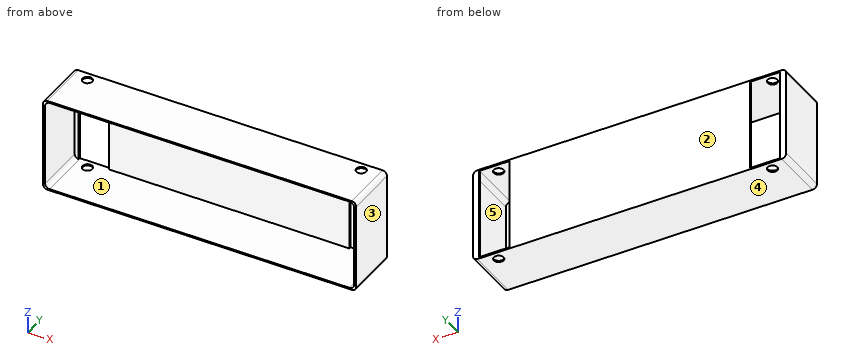
from build123d import *

# Parameters (mm, degrees)
SALIENTE_EXTRUIR1_DEPTH = 60
CROQUIS3_W              = 268.6
CROQUIS3_H              = 105
SALIENTE_EXTRUIR4_DEPTH = 2.4
CROQUIS4_R              = 5.5
CORTAR_EXTRUIR1_DEPTH   = 106


with BuildPart() as part:
    # Croquis2 → Saliente-Extruir1 (new body)
    with BuildSketch(Plane(origin=(0, 0, 0), x_dir=(1, 0, 0), z_dir=(0, 1, 0))):
        with BuildLine():
            Line((-170, 52.5), (170, 52.5))
            ThreePointArc((170, 52.5), (173.535533906, 51.035533906), (175, 47.5))
            Line((175, 47.5), (175, -47.5))
            ThreePointArc((175, -47.5), (173.535533906, -51.035533906), (170, -52.5))
            Line((170, -52.5), (-170, -52.5))
            ThreePointArc((-170, -52.5), (-173.535533906, -51.035533906), (-175, -47.5))
            Line((-175, -47.5), (-175, 47.5))
            ThreePointArc((-175, 47.5), (-173.535533906, 51.035533906), (-170, 52.5))
        make_face()
        with BuildLine():
            Line((-167.6, 51), (167.6, 51))
            ThreePointArc((167.6, 51), (171.135533906, 49.535533906), (172.6, 46))
            Line((172.6, 46), (172.6, -46))
            ThreePointArc((172.6, -46), (171.135533906, -49.535533906), (167.6, -51))
            Line((167.6, -51), (-167.6, -51))
            ThreePointArc((-167.6, -51), (-171.135533906, -49.535533906), (-172.6, -46))
            Line((-172.6, -46), (-172.6, 46))
            ThreePointArc((-172.6, 46), (-171.135533906, 49.535533906), (-167.6, 51))
        make_face(mode=Mode.SUBTRACT)
    extrude(amount=SALIENTE_EXTRUIR1_DEPTH)

    # Croquis3 → Saliente-Extruir4 (add)
    with BuildSketch(Plane(origin=(0, 60, 0), x_dir=(1, 0, 0), z_dir=(0, 1, 0))):
        with BuildLine():
            Line((-170, 52.5), (-168.3, 52.5))
            Line((-168.3, 52.5), (-168.3, -52.5))
            Line((-168.3, -52.5), (-170, -52.5))
            ThreePointArc((-170, -52.5), (-173.535533906, -51.035533906), (-175, -47.5))
            Line((-175, -47.5), (-175, 47.5))
            ThreePointArc((-175, 47.5), (-173.535533906, 51.035533906), (-170, 52.5))
        make_face()
        with BuildLine():
            Line((170, 52.5), (168.3, 52.5))
            Line((168.3, 52.5), (168.3, -52.5))
            Line((168.3, -52.5), (170, -52.5))
            ThreePointArc((170, -52.5), (173.535533906, -51.035533906), (175, -47.5))
            Line((175, -47.5), (175, 47.5))
            ThreePointArc((175, 47.5), (173.535533906, 51.035533906), (170, 52.5))
        make_face()
        Rectangle(CROQUIS3_W, CROQUIS3_H)
    extrude(amount=-SALIENTE_EXTRUIR4_DEPTH)

    # Croquis4 → Cortar-Extruir1 (cut, through all)
    with BuildSketch(Plane.XY.offset(52.5)):
        with Locations((152, 50)):
            Circle(CROQUIS4_R)
        with Locations((-154, 50)):
            Circle(CROQUIS4_R)
    extrude(amount=-CORTAR_EXTRUIR1_DEPTH, mode=Mode.SUBTRACT)


solid = part.part
For this review, take the finished solid that the model builds, in its own axes (mm). Face numbers are marked on the shaded views. A direction names the side the tool comes from. Give positions to 0.01 mm unless a question says otherwise; leave off trailing zeros. Order: outer loops, then holes, each group sorted by start corner. A loop starts at its lowest first (then second) coordinate and runs counter-clockwise, first axis right, second up. Notation, with made-up numbers: M 56,-36 L 74,-36 A32 cw 74,-8 Z; hole C 86.25,-10.75 d7. An arc over 180 degrees is marked long. Answer in a Markdown table with one row per item. Add a question column.
(1) Consider section A-A on y = 50. Give the number of separate pieces and of enclosed holes in the cut face, and give its area (3 significant figures).
(2) Consider section D-D on x = 10. State the section outline as (y, z) points.
(3) Wall thickness on probe 1 along Y at (x, z) = (-154, -51.95); probe 2 along Z at (x, y) = (150, 42); probe 3 along X at (y, z) = (53, 23): over which ranges is each line inside the solid? List them lowest first. Write a range as [from, to].
(4) Consider section B-B on x = 152. State the section outline as (y, z) points, and give its area (3 significant figures).
(5) Consider section C-C on z = 4. State the section outline as (x, y) points.
(6) Mouldability with a two-part tool opening along Z and no side actions: class the marked faces 3, 4 and 5 as +Z half, -Z half, draft (parallel to the pull), parting line (faces both ways), or undercut.
(7) For the marked faces 1 and 2, list the 3-axis set-ups (+Z, -Z, +X, -X, +Y, -Y) from which the entire face can be reached by the end or side of a thin tool; tool diameter is ignored.
(8) For pin 1 (4.5 mm diameter, centred on x = 169.5, z = 15, fed in from -Y); pin 2 (3.5 mm diameter, centred on x = -171.5, z = -1.5, fed in from -Y); pin 3 (6.5 mm diameter, centred on x = 152, y = 50, fed in from +Z), all flat-tipped, find the tip position at first contact; note any pin that passes through.
Evaluation:
| question | item | result |
|---|---|---|
| 1 | separate pieces | 4 |
| 1 | enclosed holes | 0 |
| 1 | area | 1,470 mm^2 |
| 2 | outline | M 0,-52.5 L 60,-52.5 L 60,52.5 L 0,52.5 L 0,51 L 57.6,51 L 57.6,-51 L 0,-51 Z |
| 3 | probe 1 | y = [0, 44.5], [55.5, 60] |
| 3 | probe 2 | z = [-52.5, -51], [51, 52.5] |
| 3 | probe 3 | x = [-175, -172.6], [172.6, 175] |
| 4 | outline | M 0,-52.5 L 44.5,-52.5 L 44.5,-51 L 0,-51 Z; M 0,51 L 44.5,51 L 44.5,52.5 L 0,52.5 Z; M 55.5,-52.5 L 60,-52.5 L 60,-51 L 55.5,-51 Z; M 55.5,51 L 60,51 L 60,52.5 L 55.5,52.5 Z |
| 4 | area | 147 mm^2 |
| 5 | outline | M -175,0 L -172.6,0 L -172.6,57.6 L -168.3,57.6 L -168.3,60 L -175,60 Z; M -134.3,57.6 L 134.3,57.6 L 134.3,60 L -134.3,60 Z; M 168.3,57.6 L 172.6,57.6 L 172.6,0 L 175,0 L 175,60 L 168.3,60 Z |
| 6 | face 3 | draft |
| 6 | face 4 | -Z half |
| 6 | face 5 | undercut |
| 7 | face 1 | -Y |
| 7 | face 2 | +Z, -Z, +X, -X, +Y |
| 8 | pin 1 | stops at y = 57.6 |
| 8 | pin 2 | stops at y = 0 |
| 8 | pin 3 | passes through |
